The listing builds one solid part. Answer for the finished solid, in the listing's coordinates (mm). A direction names the side the tool comes from. Round coordinates to 2 decimals unless told otherwise and drop trailing zeros. Write each loop counter-clockwise with the first axis right and the second up, starting at its lowest first coordinate (ties: lowest second). Pieces come first, ordered by that corner, then holes. Notation, with made-up numbers: (85, -13.75) - (109, -13.75) arc R33 cw to (109, 24.25) - close; hole circle Ø8 at (-6.5, -38.75). An arc over 180 degrees is marked (long way). Answer as CSV lines item,"result". Start each with the question number.
Item 1: Which of the six approach directions +Z, -Z, +X, -X, +Y, -Y give full straight-line access (tool end or side, diameter ignored) to faces 4 (the flat face through (15, 30, 5)), 5 (the flat face through (3, 15, 6.2)), 6 (the cylindrical face through (14.731, 27.747, 2.636))?
Item 2: A cutting plane is placed at C-C on x = 15. Determine the outline of the cut face in (y, z), and give its area (3 significant figures).
Item 3: Straight lines are drawn through the part: line 1 along X through (y, z) = (2, 8.55); line 2 along X through (y, z) = (2, 2); line 3 along Y through (x, z) = (15, 8.5). For each, find the intervals that lie inside material, in ascending order. Write a range as [from, to].
Item 4: A cutting plane is placed at B-B on z = 3.75. Determine the outline of the cut face in (x, y).
Item 5: Flat-ended cylindrical pins translate along their axes: pin 1 (1.8 mm diameter, centred on y = 10.5, z = 7.5, fed in from -X); pin 2 (3 mm diameter, centred on x = 23.5, y = 20.5, fed in from -Z). Find the tip coordinate at first contact, or state that the pin passes through.
Item 6: A cutting plane is placed at D-D on y = 14.5. Determine the outline of the cut face in (x, z), and give its area (3 significant figures).
Item 7: A cutting plane is placed at A-A on y = 2. Determine the outline of the cut face in (x, z).
Item 8: For a pull along X with two mould halves and no side action, classify faces 1 (the flat face through (27.25, 8, 3)), 2 (the flat face through (0, 15, 5)), 3 (the flat face through (14, 0, 9)) as pulls with the +X half, pulls with the -X half, needs draft (parallel to the pull), parting line crosses it, or undercut.
```python
from build123d import *

# Parameters (mm, degrees)
ESQUISSE1_W                                       = 30
ESQUISSE1_H                                       = 30
MAIN_DEPTH                                        = 10
MAIN_FIX_DEPTH                                    = 28.5
BOSS_EXTRU_2_DEPTH                                = 8.4
BOSS_EXTRU_3_DEPTH                                = 1
FRAISAGE_POUR_VIS_T_TE_FRAIS_E_BOMB_E_D           = 2.5999948
FRAISAGE_POUR_VIS_T_TE_FRAIS_E_BOMB_E_CSINK_D     = 5.0546
FRAISAGE_POUR_VIS_T_TE_FRAIS_E_BOMB_E_CSINK_ANGLE = 82


with BuildPart() as part:
    # Esquisse1 → Main (new body)
    with BuildSketch(Plane.XY):
        with Locations((15, 15)):
            Rectangle(ESQUISSE1_W, ESQUISSE1_H)
    extrude(amount=MAIN_DEPTH)

    # Esquisse2 → Main Fix (cut)
    with BuildSketch(Plane.XZ):
        Polygon((2.75, 0), (2.75, 5.2), (3.35, 5.2), (3.35, 6.2), (2.75, 6.2), (2.75, 8.4), (27.25, 8.4), (27.25, 6.2), (26.65, 6.2), (26.65, 5.2), (27.25, 5.2), (27.25, 0), align=None)
    extrude(amount=-MAIN_FIX_DEPTH, mode=Mode.SUBTRACT)

    # Esquisse4 → Boss.-Extru.2 (add)
    with BuildSketch(Plane(origin=(0, 0, 8.4), x_dir=(-1, 0, 0), z_dir=(0, 0, -1))):
        with BuildLine():
            Line((-27.25, 15.5), (-27.25, 28.5))
            Line((-27.25, 28.5), (-2.75, 28.5))
            Line((-2.75, 28.5), (-2.75, 15.5))
            ThreePointArc((-2.75, 15.5), (-15, 27.75), (-27.25, 15.5))
        make_face()
    extrude(amount=BOSS_EXTRU_2_DEPTH)

    # Esquisse5 → Boss.-Extru.3 (add)
    with BuildSketch(Plane(origin=(0, 0, 5.2), x_dir=(-1, 0, 0), z_dir=(0, 0, -1))):
        with BuildLine():
            Line((-3.35, 13.970294146), (0, 13.970294146))
            Line((0, 13.970294146), (0, 30))
            Line((0, 30), (-30, 30))
            Line((-30, 30), (-30, 13.970294146))
            Line((-30, 13.970294146), (-26.65, 13.970294146))
            ThreePointArc((-26.65, 13.970294146), (-15, 27.25), (-3.35, 13.970294146))
        make_face()
    extrude(amount=-BOSS_EXTRU_3_DEPTH)

    # Fraisage pour vis à tête fraisée bombée #33 (through all)
    with Locations(Plane.XY.offset(10)):
        with Locations((15, 2)):
            CounterSinkHole(FRAISAGE_POUR_VIS_T_TE_FRAIS_E_BOMB_E_D / 2, FRAISAGE_POUR_VIS_T_TE_FRAIS_E_BOMB_E_CSINK_D / 2, counter_sink_angle=FRAISAGE_POUR_VIS_T_TE_FRAIS_E_BOMB_E_CSINK_ANGLE)


solid = part.part
```
Geometry says:
1,face 4,"+Z, -Z, +X, -X, +Y"
1,face 5,"-Y"
1,face 6,"-Z, -Y"
2,outline,"(0, 8.4) - (0.7, 8.4) - (0.7, 8.59) - (0, 9.39) - close; (3.3, 8.4) - (27.75, 8.4) - (27.75, 6.2) - (27.25, 6.2) - (27.25, 5.2) - (27.75, 5.2) - (27.75, 0) - (30, 0) - (30, 10) - (4.53, 10) - (3.3, 8.59) - close"
2,area,"61.7 mm^2"
3,line 1,"x = [0, 13.7], [16.3, 30]"
3,line 2,"x = [0, 2.75], [27.25, 30]"
3,line 3,"y = [0, 0.7], [3.3, 30]"
4,outline,"(0, 0) - (2.75, 0) - (2.75, 15.5) arc R12.25 cw to (27.25, 15.5) - (27.25, 0) - (30, 0) - (30, 30) - (0, 30) - close"
5,pin 1,"stops at x = 0"
5,pin 2,"stops at z = 8.4"
6,outline,"(0, 0) - (2.75, 0) - (2.75, 5.2) - (3.35, 5.2) - (3.35, 6.2) - (2.75, 6.2) - (2.75, 8.4) - (27.25, 8.4) - (27.25, 6.2) - (26.65, 6.2) - (26.65, 5.2) - (27.25, 5.2) - (27.25, 0) - (30, 0) - (30, 10) - (0, 10) - close"
6,area,"95.4 mm^2"
7,outline,"(0, 0) - (2.75, 0) - (2.75, 5.2) - (3.35, 5.2) - (3.35, 6.2) - (2.75, 6.2) - (2.75, 8.4) - (13.7, 8.4) - (13.7, 8.59) - (12.47, 10) - (0, 10) - close; (16.3, 8.4) - (27.25, 8.4) - (27.25, 6.2) - (26.65, 6.2) - (26.65, 5.2) - (27.25, 5.2) - (27.25, 0) - (30, 0) - (30, 10) - (17.53, 10) - (16.3, 8.59) - close"
8,face 1,"undercut"
8,face 2,"pulls with the -X half"
8,face 3,"needs draft"
